```python
from build123d import *

# Parameters (mm, degrees)
PAD_DEPTH = 18


with BuildPart() as part:
    # Sketch → Pad (new body)
    with BuildSketch(Plane.XZ):
        with BuildLine():
            Line((-170, 0), (170, 0))
            Line((170, 0), (170, 380))
            Line((170, 380), (90, 380))
            ThreePointArc((-90, 380), (0, 350), (90, 380))
            Line((-90, 380), (-170, 380))
            Line((-170, 380), (-170, 0))
        make_face()
    extrude(amount=PAD_DEPTH)


solid = part.part
```
Could you check a few things on this model? Use its own coordinates, in mm. Coordinates: 2 decimals unless noted, no trailing zeros. Order: outer loops, then holes, each group sorted by start corner. A loop starts at its lowest first (then second) coordinate and runs counter-clockwise, first axis right, second up. Notation, with made-up numbers: M -24,16.25 L 16,16.25 A17 cw 16,24.25 Z; hole C 73,20 d8. An arc over 180 degrees is marked long. Use one line per item in the form item = value. Start each with the question number.
1. Suppose I cut it at D-D on x = -19.5. Write out the boundary of the cut face in (y, z), then the cut area to 3 significant figures.
2. Suppose I cut it at A-A on z = 357. Write out the boundary of the cut face in (x, y).
3. Please list where these lines run through material, in increasing order: line 1 (X direction, y = -15.5, z = 361); line 2 (Z direction, x = -28, y = -4); line 3 (Z direction, x = -37.5, y = -6.25).
4. For pin 1 (10 mm diameter, centred on x = 81.5, y = -7.5, fed in from +Z), with a flat end and sliding along its axis, tell me the tip position at first contact or that it passes through.
5. We'd pull the mould along X, two halves only. Please class faces 1 (the flat face through (170, -9, 187)), 2 (the cylindrical face through (-1.351, -8.874, 350.006)), 3 (the flat face through (131, -9, 380)): +X half, -X half, draft (parallel to the pull), parting line (faces both ways), or undercut.
6. Suppose I cut it at B-B on y = -7.75. Write out the boundary of the cut face in (x, z), then the cut area to 3 significant figures.
7. Suppose I cut it at C-C on x = 78. Write out the boundary of the cut face in (y, z).
Geometry says:
q1.outline = M -18,0 L 0,0 L 0,351.27 L -18,351.27 Z
q1.area = 6,320 mm^2
q2.outline = M -170,-18 L -45.29,-18 L -45.29,0 L -170,0 Z; M 45.29,-18 L 170,-18 L 170,0 L 45.29,0 Z
q3.line_1 = -170 to -56.38, 56.38 to 170
q3.line_2 = 0 to 352.64
q3.line_3 = 0 to 354.76
q4.pin_1 = 377.45
q5.face_1 = +X half
q5.face_2 = undercut
q5.face_3 = draft
q6.outline = M -170,0 L 170,0 L 170,380 L 90,380 A150 cw -90,380 L -170,380 Z
q6.area = 126,000 mm^2
q7.outline = M -18,0 L 0,0 L 0,371.88 L -18,371.88 Z
